For this review, take the finished solid that the model builds, in its own axes (mm). Round coordinates to 2 decimals unless told otherwise and drop trailing zeros. Order: outer loops, then holes, each group sorted by start corner. A loop starts at its lowest first (then second) coordinate and runs counter-clockwise, first axis right, second up. Notation, with made-up numbers: M 87.5,-31.5 L 124.5,-31.5 A14 ccw 124.5,-27.5 Z; hole C 77.25,15 d3. An arc over 180 degrees is marked long. Answer in a Markdown table with one row per item. Add a question column.
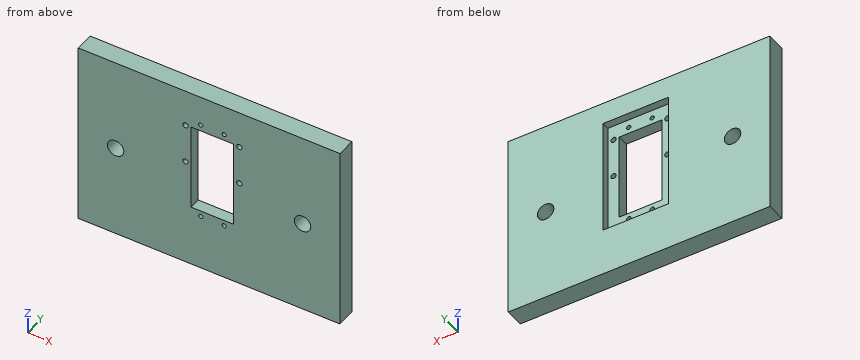
```python
from build123d import *

# Parameters (mm, degrees)
SKETCH1_W           = 177.8
SKETCH1_H           = 127
SKETCH1_R           = 5.588
SKETCH1_R_2         = 1.8288
SKETCH1_R_3         = 1.4605
SKETCH1_W_2         = 28.956
SKETCH1_H_2         = 59.69
BOSS_EXTRUDE1_DEPTH = 12.7
SKETCH2_W           = 44.45
SKETCH2_H           = 79.4004
CUT_EXTRUDE1_DEPTH  = 5.08


with BuildPart() as part:
    # Sketch1 → Boss-Extrude1 (new body)
    with BuildSketch(Plane(origin=(0, 0, 0), x_dir=(1, 0, 0), z_dir=(0, 1, 0))):
        Rectangle(SKETCH1_W, SKETCH1_H)
        with Locations((-63.5, 0)):
            Circle(SKETCH1_R, mode=Mode.SUBTRACT)
        with Locations((63.5, 0)):
            Circle(SKETCH1_R, mode=Mode.SUBTRACT)
        with Locations((20.557934463, -38.085909964)):
            Circle(SKETCH1_R_2, mode=Mode.SUBTRACT)
        with Locations((-16.018065537, -38.085909964)):
            Circle(SKETCH1_R_2, mode=Mode.SUBTRACT)
        with Locations((-16.018065537, -11.145141601)):
            Circle(SKETCH1_R_2, mode=Mode.SUBTRACT)
        with Locations((20.557934463, -11.145141601)):
            Circle(SKETCH1_R_2, mode=Mode.SUBTRACT)
        with Locations((-5.667565537, -42.871775783)):
            Circle(SKETCH1_R_3, mode=Mode.SUBTRACT)
        with Locations((10.207434463, -42.871775783)):
            Circle(SKETCH1_R_3, mode=Mode.SUBTRACT)
        with Locations((-5.667565537, 25.149424217)):
            Circle(SKETCH1_R_3, mode=Mode.SUBTRACT)
        with Locations((10.207434463, 25.149424217)):
            Circle(SKETCH1_R_3, mode=Mode.SUBTRACT)
        with Locations((2.269934463, -8.661150783)):
            Rectangle(SKETCH1_W_2, SKETCH1_H_2, mode=Mode.SUBTRACT)
    extrude(amount=BOSS_EXTRUDE1_DEPTH)

    # Sketch2 → Cut-Extrude1 (cut)
    with BuildSketch(Plane(origin=(0, 12.7, 0), x_dir=(1, 0, 0), z_dir=(0, 1, 0))):
        with Locations((2.269934463, -8.737350783)):
            Rectangle(SKETCH2_W, SKETCH2_H)
    extrude(amount=-CUT_EXTRUDE1_DEPTH, mode=Mode.SUBTRACT)


solid = part.part
```
1. Consider section B-B on z = 0. Write out the cut boundary in (x, y).
2. Clearance check with flat-ended pins moving along their axes: pin 1 Ø4 at (x, z) = (10.21, 42.87) entering from -Y; pin 2 Ø3 at (x, z) = (20.56, 11.15) entering from -Y; pin 3 Ø5 at (x, z) = (-16.02, 11.15) entering from +Y. State where each tip first meets the part, or that it passes through.
3. To check wall thickness, follow probe 1 along X at (y, z) = (3, -9); probe 2 along Z at (x, y) = (-14, 11); probe 3 along X at (y, z) = (10, 9.5). State the ranges of each line that lie inside material, in increasing order. Write a range as [from, to].
4. Consider section A-A on x = 63.5. Write out the cut boundary in (y, z), plus the area to 3 significant figures.
5. Consider section C-C on y = 5.5. State how many separate pieces and enclosed holes the cut face has, plus the area to 3 significant figures.
Solved:
| question | item | result |
|---|---|---|
| 1 | outline | M -88.9,0 L -69.09,0 L -69.09,12.7 L -88.9,12.7 Z; M -57.91,0 L -12.21,0 L -12.21,7.62 L -19.96,7.62 L -19.96,12.7 L -57.91,12.7 Z; M 16.75,0 L 57.91,0 L 57.91,12.7 L 24.49,12.7 L 24.49,7.62 L 16.75,7.62 Z; M 69.09,0 L 88.9,0 L 88.9,12.7 L 69.09,12.7 Z |
| 2 | pin 1 | stops at y = 0 |
| 2 | pin 2 | passes through |
| 2 | pin 3 | stops at y = 7.62 |
| 3 | probe 1 | x = [-88.9, -12.21], [16.75, 88.9] |
| 3 | probe 2 | z = [-63.5, -30.96], [48.44, 63.5] |
| 3 | probe 3 | x = [-88.9, -19.96], [24.49, 88.9] |
| 4 | outline | M 0,-63.5 L 12.7,-63.5 L 12.7,-5.59 L 0,-5.59 Z; M 0,5.59 L 12.7,5.59 L 12.7,63.5 L 0,63.5 Z |
| 4 | area | 1,470 mm^2 |
| 5 | separate pieces | 1 |
| 5 | enclosed holes | 11 |
| 5 | area | 20,600 mm^2 |
